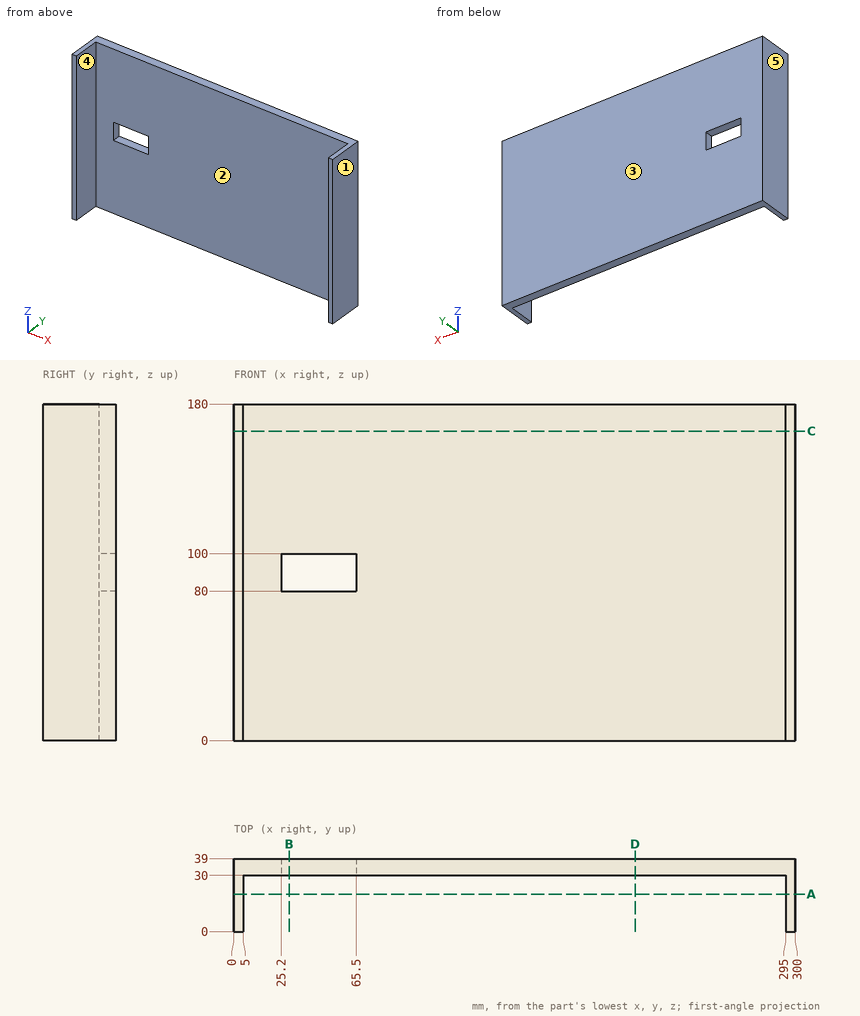
For this review, use the dimensioned drawing (mm, ordinates from the lowest corner) and the shaded views. A direction names the side the tool comes from. Give positions to 0.01 mm unless a question says otherwise; leave off trailing zeros. Loops run counter-clockwise (first coordinate to the right, second up) from the corner with the lowest first, then second, coordinate; pieces in that order, holes last.
Item 1: Take a section at D-D, the plane x = 214.5. State the section outline as (y, z) points.
Item 2: Take a section at B-B, the plane x = 29.5. State the section outline as (y, z) points, and give its area (3 significant figures).
Item 3: Take a section at C-C, the plane z = 165.5. State the section outline as (x, y) points, and give its area (3 significant figures).
Item 4: Draft analysis for pull direction X (two halves, no side actions). For the marked faces 1, 2 and 3, state which applies: +X half, -X half, draft (parallel to the pull), parting line (faces both ways), or undercut.
Item 5: Take a section at A-A, the plane y = 20. State the section outline as (x, z) points, and give its area (3 significant figures).
Item 6: Tool access review of the marked faces 4 and 5: name each direction out of +Z, -Z, +X, -X, +Y, -Y from which nothing blocks a thin tool from reaching the whole face with its end or side.
Item 7: Insertion check: pin 1 (7 mm diameter, centred on x = 53, y = 35.5, fed in from -Z); pin 2 (4 mm diameter, centred on x = 55.5, z = 122.5, fed in from -Y). Each pin has a flat end and moves straight along its axis. Give the tip position at first contact, or say it passes through.
Item 8: For line 1 along X through (y, z) = (10.5, 100.5); line 2 along Y through (x, z) = (210, 79), list the stretches that pass through material, from the lowest coordinate up.
Calculated:
1. outline: (30, 0) - (39, 0) - (39, 180) - (30, 180) - close
2. outline: (30, 0) - (39, 0) - (39, 80) - (30, 80) - close; (30, 100) - (39, 100) - (39, 180) - (30, 180) - close
2. area: 1,440 mm2
3. outline: (0, 0) - (5, 0) - (5, 30) - (295, 30) - (295, 0) - (300, 0) - (300, 39) - (0, 39) - close
3. area: 3,000 mm2
4. face 1: +X half
4. face 2: undercut
4. face 3: draft
5. outline: (0, 0) - (5, 0) - (5, 180) - (0, 180) - close; (295, 0) - (300, 0) - (300, 180) - (295, 180) - close
5. area: 1,800 mm2
6. face 4: +Z, -Z, -Y
6. face 5: +Z, -Z, -X, +Y, -Y
7. pin 1: stops at z = 0
7. pin 2: stops at y = 30
8. line 1: x = 0 to 5, 295 to 300
8. line 2: y = 30 to 39
